from build123d import *

# Parameters (mm, degrees)
SKETCH2_R               = 7.5
SKETCH2_R_2             = 2.65
BOSS_EXTRUDE1_DEPTH     = 5
BOSS_EXTRUDE2_DEPTH     = 5
SKETCH4_R               = 2.5
BOSS_EXTRUDE3_DEPTH     = 45
BOSS_EXTRUDE4_DEPTH     = 5
CUT_EXTRUDE1_DEPTH      = 116.323136372
CUT_EXTRUDE1_DEPTH_BACK = 116.323136372
SKETCH6_R               = 2.15
SKETCH7_R               = 4.088958129
CUT_EXTRUDE2_DEPTH      = 1.2


with BuildPart() as part:
    # Sketch2 → Boss-Extrude1 (new body)
    with BuildSketch(Plane.ZY.offset(-18.504809472)):
        with Locations((-0.354303453, 100.78821716)):
            Circle(SKETCH2_R)
        with Locations((-0.354303453, 100.78821716)):
            Circle(SKETCH2_R_2, mode=Mode.SUBTRACT)
    extrude(amount=-BOSS_EXTRUDE1_DEPTH)

    # Sketch3 → Boss-Extrude2 (add)
    with BuildSketch(Plane.ZY.offset(-18.504809472)):
        Polygon((-9.150423673, 96.891429681), (-7.602645922, 102.714750693), (0.936612358, 94.575063583), (3.681899885, 94.466899053), (7.922814088, 89.804236476), (0.729824207, 83.261868795), (-9.719499705, 94.750351991), align=None)
    extrude(amount=-BOSS_EXTRUDE2_DEPTH)

    # Sketch4 → Boss-Extrude3 (add)
    with BuildSketch(Plane(origin=(0, 45.202809873, -41.114113503), x_dir=(1, 0, 0), z_dir=(0, -0.7397718400154494, 0.6728578042351567))):
        with Locations(Location((21.004809472, 61.424928866, 0), (0, 0, 180))):
            Circle(SKETCH4_R)
    extrude(amount=BOSS_EXTRUDE3_DEPTH)

    # Sketch5 → Boss-Extrude4 (add)
    with BuildSketch(Plane.ZY.offset(-18.504809472)):
        with BuildLine():
            Line((39.189983074, 48.290417188), (37.112992328, 55.268407542))
            Line((37.112992328, 55.268407542), (33.049229829, 59.736301118))
            Line((33.049229829, 59.736301118), (28.184844411, 55.311910361))
            Line((28.184844411, 55.311910361), (32.423819526, 50.65137971))
            Line((32.423819526, 50.65137971), (31.912552769, 47.90776949))
            ThreePointArc((31.912552769, 47.90776949), (35.794247616, 43.477955415), (39.189983074, 48.290417188))
        make_face()
    extrude(amount=-BOSS_EXTRUDE4_DEPTH)

    # Sketch6 → Cut-Extrude1 (cut, two sides: drawn at the far end of the back side and taken through both)
    with BuildSketch(Plane(origin=(23.504809472, 0, 0), x_dir=(0, 0, -1), z_dir=(1, 0, 0)).offset(-CUT_EXTRUDE1_DEPTH_BACK)):
        with Locations((-35.597432924, 47.221098797)):
            Circle(SKETCH6_R)
    extrude(amount=CUT_EXTRUDE1_DEPTH + CUT_EXTRUDE1_DEPTH_BACK, mode=Mode.SUBTRACT)

    # Sketch7 → Cut-Extrude2 (cut, symmetric)
    with BuildSketch(Plane(origin=(21.004809472, 0, 0), x_dir=(0, 0, -1), z_dir=(1, 0, 0))):
        with Locations((-35.597432924, 47.221098797)):
            Circle(SKETCH7_R)
    extrude(amount=CUT_EXTRUDE2_DEPTH, both=True, mode=Mode.SUBTRACT)


with BuildPart() as part_1:
    # Body-Move/Copy1: moved
    add(part.part.moved(Location((-21, -100.79, 0.35))))


solid = part_1.part
Input: part model. Units: mm. Frame: model coordinates. A direction names the side the tool comes from. Coordinates: 2 decimals unless noted, no trailing zeros. Loops run counter-clockwise (first coordinate to the right, second up) from the corner with the lowest first, then second, coordinate; pieces in that order, holes last. Notation, with made-up numbers: (-8.5, -17.5) -> (6.5, -17.5) arc R30 cw to (6.5, 19.5) -> close; hole circle Ø10 at (20.25, 13). An arc over 180 degrees is marked (long way). One line per item, written item: value.
(1) Cut plane C-C (y = -5). Output: boundary loops of the cut face in (x, z).
Answer below:
outline: (-2.5, -9.09) -> (2.5, -9.09) -> (2.5, 5.59) -> (-2.5, 5.59) -> close
(2) Cut plane A-A (x = -0.2). Output: boundary loops of the cut face in (y, z).
Answer below:
outline: (-51.28, 32.56) -> (-50.14, 32.77) -> (-45.48, 28.53) -> (-44.9, 29.18) -> (-15.93, 2.83) -> (-17.53, 1.08) -> (-6.04, -9.37) -> (1.92, -7.25) arc R7.5 ccw (long way) to (-6.32, 4.03) -> (-10.99, 8.27) -> (-12.58, 6.52) -> (-41.54, 32.86) -> (-41.05, 33.4) -> (-45.52, 37.46) -> (-50.93, 39.07) arc R4.09 cw to start; hole circle Ø5.3 at (0, 0)
(3) Cut plane B-B (z = 36.5). Output: boundary loops of the cut face in (x, y), then the cut area to 3 significant figures.
Answer below:
outline: (-2.5, -57.28) -> (-1.2, -57.28) -> (-1.2, -55.65) -> (-2.5, -55.65) -> close; (-2.5, -51.49) -> (-1.2, -51.49) -> (-1.2, -49.52) -> (1.2, -49.52) -> (1.2, -51.49) -> (2.5, -51.49) -> (2.5, -44.46) -> (-2.5, -44.46) -> close; (1.2, -57.28) -> (2.5, -57.28) -> (2.5, -55.65) -> (1.2, -55.65) -> close
area: 34.6 mm2
(4) Set-up query: faces 1 (the face through (-0.03, -8.62, 6.12)), 2 (the face through (-0.03, -11.87, 7.3)), 3 (the face through (-0.03, -41.4, 33.02)), 4 (the face through (2.505, -49, 34)), 5 (the face through (0.02, -49.49, 35.68)). Return all of +Z, -Z, +X, -X, +Y, -Y with unobstructed straight access to the full face (end or side cutting, diameter ignored); none if empty.
Answer below:
face 1: +Z, +X, -X
face 2: +Z
face 3: +Y
face 4: +Z, -Z, +X, +Y, -Y
face 5: -Y
(5) Draft query along Y for faces 6 (the face through (-0.03, -45.086, 28.966)), 7 (the face through (-0.03, -49.059, 38.516)), 8 (the face through (-0.03, 5.931, 4.584)), 9 (the face through (-2.495, -49, 34)). Return one class per face: pulls with the +Y half, pulls with the -Y half, needs draft (parallel to the pull), parting line crosses it, or undercut.
Answer below:
face 6: undercut
face 7: pulls with the +Y half
face 8: undercut
face 9: needs draft
(6) Ray query, line 1 along X through (y, z) = (-50.5, 37.5); line 2 along Z through (x, y) = (2, -52); line 3 along Z through (x, y) = (1.35, -2). Return the intervals inside material, ascending.
Answer below:
line 1: x = -2.5 to -1.2, 1.2 to 2.5
line 2: z = 32.43 to 34.48, 37.42 to 39.39
line 3: z = -8.3 to -1.74, 1.74 to 7.22
(7) Pin query (flat end, axial travel): pin 1 Ø2 at (x, y) = (-1, -46.5) entering from +Z; pin 2 Ø1 at (x, z) = (-1, 31.5) entering from -Y; pin 3 Ø1.5 at (x, y) = (1, -18) entering from -Z; pin 4 Ø5.5 at (y, z) = (-53.57, 35.95) entering from +X. Return the tip coordinate at first contact, or that it passes through.
Answer below:
pin 1: stops at z = 38.05
pin 2: stops at y = -49.29
pin 3: stops at z = 0.83
pin 4: stops at x = 2.5
